Build history of the part. All positions in model axes, mm. A direction names the side the tool comes from. Coordinates: 2 decimals unless noted, no trailing zeros. Loops run counter-clockwise (first coordinate to the right, second up) from the corner with the lowest first, then second, coordinate; pieces in that order, holes last. Notation, with made-up numbers: (46.5, -38.75) -> (65.5, -38.75) arc R21 cw to (65.5, -7.75) -> close; hole circle Ø10 at (35, 49). An arc over 180 degrees is marked (long way). One line per item, written item: value. Start each with the question number.
```python
from build123d import *

# Parameters (mm, degrees)
F0_R          = 60
F0_R_2        = 30
F1_DEPTH      = 1000
F3_R          = 15
F4_DEPTH      = 100
F4_DEPTH_BACK = 7
F6_R          = 15
F7_DEPTH      = 100
F7_DEPTH_BACK = 7


with BuildPart() as f1:
    # F0 (on Front) → F1 (new body)
    with BuildSketch(Plane.XZ):
        Circle(F0_R)
        Circle(F0_R_2, mode=Mode.SUBTRACT)
    extrude(amount=F1_DEPTH)

    # F3 (on offset) → F4 (join, two sides)
    with BuildSketch(Plane.XY.offset(60)) as f4_sk:
        with Locations((0, -15)):
            Circle(F3_R)
    extrude(amount=F4_DEPTH)
    extrude(f4_sk.sketch, amount=-F4_DEPTH_BACK)

    # F6 (on offset) → F7 (join, two sides)
    with BuildSketch(Plane.XY.offset(-60)) as f7_sk:
        with Locations((0, -980.9999256134)):
            Circle(F6_R)
    extrude(amount=-F7_DEPTH)
    extrude(f7_sk.sketch, amount=F7_DEPTH_BACK)


solid = f1.part
```
Item 1: Two-plate mould, pull along Z, no slides. Class faces 3 (the face through (-59.94, -493, 2.64)), 4 (the face through (12, -1000, 28)), 5 (the face through (0, -981, -160)), 6 (the face through (-29.97, -493, 1.32)): +Z half, -Z half, draft (parallel to the pull), parting line (faces both ways), or undercut.
Item 2: Band-saw the part on B-B, the plane y = -487.5. List the corners of the cut face in (x, z), and give its area (3 significant figures).
Item 3: Tool access for faces 1 (the face through (-1.953, -966.128, -109.76)), 2 (the face through (0, -15, 160)): list every direction of +Z, -Z, +X, -X, +Y, -Y with a clear straight run to the whole face (end or side of a thin tool).
Item 4: Band-saw the part on C-C, the plane z = 116. List the corners of the cut face in (x, y).
Item 5: Band-saw the part on A-A, the plane z = 0. List the corners of the cut face in (x, y), and give its area (3 significant figures).
Item 6: Probe probe 1 along Z at (x, y) = (0, -644); probe 2 along Z at (x, y) = (24, -380); probe 3 along Y at (x, z) = (2, -63). List the from-to ranges inside material, lowest first.
Item 7: Band-saw the part on D-D, the plane x = -48.5. List the corners of the cut face in (y, z), and give its area (3 significant figures).
Item 8: Drop flat-ended pins along their axis: pin 1 Ø10 at (x, y) = (-26, -386) entering from -Z (3 decimals); pin 2 Ø8 at (y, z) = (-369, 58.5) entering from -X; pin 3 Ø4 at (x, z) = (-8.5, 111) entering from +Y. Give the stop position or say it passes through.
Worked out:
1. face 3: parting line
1. face 4: draft
1. face 5: -Z half
1. face 6: undercut
2. outline: circle Ø120 at (0, 0); hole circle Ø60 at (0, 0)
2. area: 8,480 mm²
3. face 1: -Z
3. face 2: +Z, +X, -X, +Y, -Y
4. outline: circle Ø30 at (0, -15)
5. outline: (-60, -1000) -> (-30, -1000) -> (-30, 0) -> (-60, 0) -> close; (30, -1000) -> (60, -1000) -> (60, 0) -> (30, 0) -> close
5. area: 60,000 mm²
6. probe 1: z = -60 to -30, 30 to 60
6. probe 2: z = -54.99 to -18, 18 to 54.99
6. probe 3: y = -995.87 to -966.13
7. outline: (-1000, -35.32) -> (0, -35.32) -> (0, 35.32) -> (-1000, 35.32) -> close
7. area: 70,600 mm²
8. pin 1: stops at z = -56.205
8. pin 2: stops at x = -25.09
8. pin 3: stops at y = -1.48
